Part print with two shaded views. Sizes in mm from the minimum x, y, z corner. Give positions to 0.01 mm unless a question says otherwise; leave off trailing zeros. Order: outer loops, then holes, each group sorted by start corner. A loop starts at its lowest first (then second) coordinate and runs counter-clockwise, first axis right, second up.
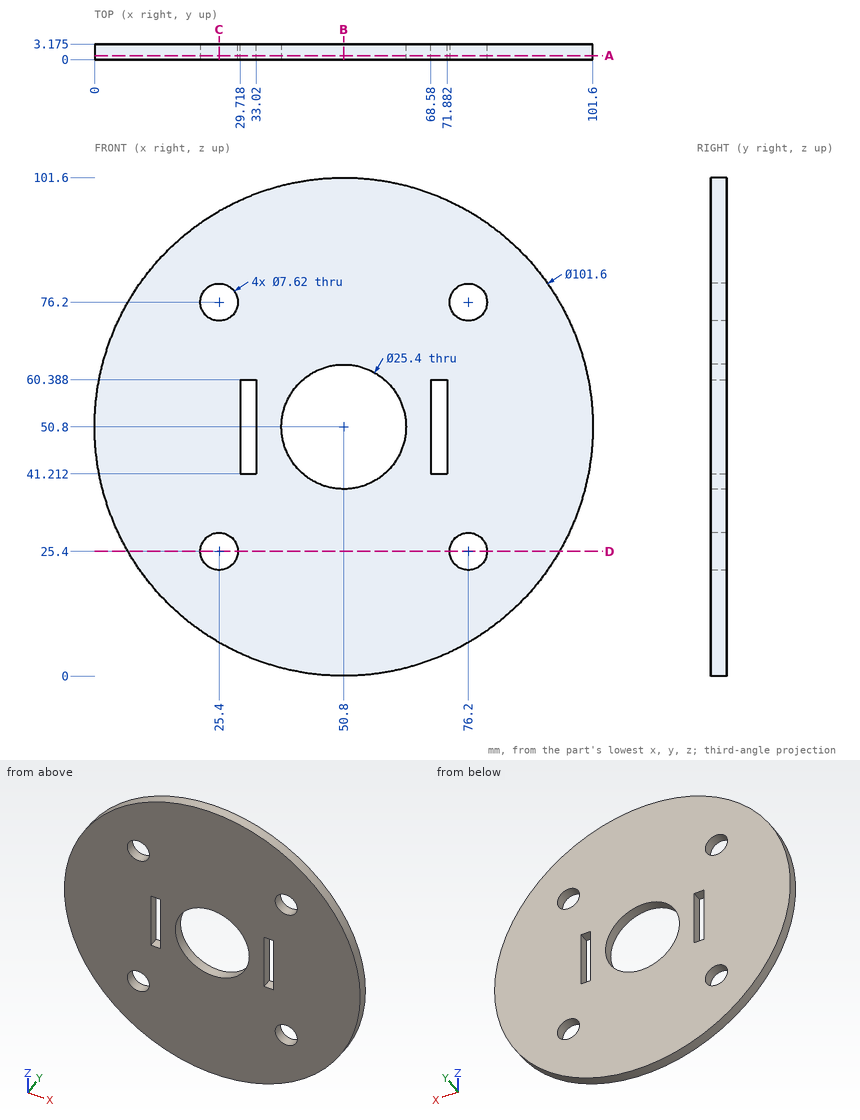
Item 1: Slice it at B-B (x = 50.8). Give the cut face in (y, z) (1 decimal).
Item 2: Slice it at A-A (y = 0.8). Give the cut face in (x, z), and give its area (3 significant figures).
Item 3: Wall check: L1, parallel to X at y = 1.1, z = 50.8; L2, parallel to Z at x = 25.4, y = 1.15 (1 decimal); L3, parallel to Z at x = 50.8, y = 1.8. Give the ranges that are in metal, low to high.
Item 4: Drop flat-ended pins along their axis: pin 1 Ø4.5 at (x, z) = (76.2, 76.2) entering from +Y; pin 2 Ø1.6 at (y, z) = (1, 52.5) entering from -X; pin 3 Ø1 at (y, z) = (1.5, 47.5) entering from +X; pin 4 Ø1 at (y, z) = (2.5, 55.5) entering from -X. Give the stop position or say it passes through.
Item 5: Slice it at D-D (z = 25.4). Give the cut face in (x, y) (1 decimal), and give its area (3 significant figures).
Item 6: Slice it at C-C (x = 25.4). Give the cut face in (y, z) (1 decimal), and give its area (3 significant figures).
A:
1. outline: (0, 0) - (3.2, 0) - (3.2, 38.1) - (0, 38.1) - close; (0, 63.5) - (3.2, 63.5) - (3.2, 101.6) - (0, 101.6) - close
2. outline: circle Ø101.6 at (50.8, 50.8); hole circle Ø7.62 at (25.4, 25.4); hole circle Ø7.62 at (25.4, 76.2); hole (29.72, 41.21) - (33.02, 41.21) - (33.02, 60.39) - (29.72, 60.39) - close; hole circle Ø25.4 at (50.8, 50.8); hole (68.58, 41.21) - (71.88, 41.21) - (71.88, 60.39) - (68.58, 60.39) - close; hole circle Ø7.62 at (76.2, 25.4); hole circle Ø7.62 at (76.2, 76.2)
2. area: 7,290 mm2
3. L1: x = 0 to 29.72, 33.02 to 38.1, 63.5 to 68.58, 71.88 to 101.6
3. L2: z = 6.8 to 21.6, 29.2 to 72.4, 80 to 94.8
3. L3: z = 0 to 38.1, 63.5 to 101.6
4. pin 1: passes through
4. pin 2: stops at x = 0.01
4. pin 3: stops at x = 101.52
4. pin 4: stops at x = 0.17
5. outline: (6.8, 0) - (21.6, 0) - (21.6, 3.2) - (6.8, 3.2) - close; (29.2, 0) - (72.4, 0) - (72.4, 3.2) - (29.2, 3.2) - close; (80, 0) - (94.8, 0) - (94.8, 3.2) - (80, 3.2) - close
5. area: 231 mm2
6. outline: (0, 6.8) - (3.2, 6.8) - (3.2, 21.6) - (0, 21.6) - close; (0, 29.2) - (3.2, 29.2) - (3.2, 72.4) - (0, 72.4) - close; (0, 80) - (3.2, 80) - (3.2, 94.8) - (0, 94.8) - close
6. area: 231 mm2
